Source: CAD feature listing. Evaluate the final solid. Frame: model axes, mm. Face numbers are marked on the shaded views. A direction names the side the tool comes from. Give positions to 0.01 mm unless a question says otherwise; leave off trailing zeros. Loops run counter-clockwise (first coordinate to the right, second up) from the corner with the lowest first, then second, coordinate; pieces in that order, holes last. Notation, with made-up numbers: (56, 28.25) - (94, 28.25) arc R28 cw to (94, 66.25) - close; hole circle Ø9 at (33.25, 81.25). An arc over 180 degrees is marked (long way). Put each result on its own line as item: value.
```python
from build123d import *

# Parameters (mm, degrees)
SKETCH1_W           = 205.38
SKETCH1_H           = 118.65
SKETCH1_W_2         = 189.38
SKETCH1_H_2         = 102.65
BOSS_EXTRUDE1_DEPTH = 13.5
SKETCH3_W           = 205.38
SKETCH3_H           = 118.65
BOSS_EXTRUDE2_DEPTH = 6.5
SKETCH4_R           = 2.5
CUT_EXTRUDE1_DEPTH  = 6
FILLET1_R           = 12.94


with BuildPart() as part:
    # Sketch1 → Boss-Extrude1 (new body)
    with BuildSketch(Plane(origin=(0, 0, 0), x_dir=(1, 0, 0), z_dir=(0, 1, 0))):
        Rectangle(SKETCH1_W, SKETCH1_H)
        Rectangle(SKETCH1_W_2, SKETCH1_H_2, mode=Mode.SUBTRACT)
    extrude(amount=BOSS_EXTRUDE1_DEPTH)

    # Sketch3 → Boss-Extrude2 (add)
    with BuildSketch(Plane(origin=(0, 13.5, 0), x_dir=(1, 0, 0), z_dir=(0, 1, 0))):
        Rectangle(SKETCH3_W, SKETCH3_H)
        Polygon((-94.69, 31.325), (-74.69, 51.325), (74.69, 51.325), (94.69, 31.325), (94.69, -31.325), (74.69, -51.325), (-74.69, -51.325), (-94.69, -31.325), align=None, mode=Mode.SUBTRACT)
    extrude(amount=BOSS_EXTRUDE2_DEPTH)

    # Sketch4 → Cut-Extrude1 (cut)
    with BuildSketch(Plane.XZ.offset(-13.5)):
        with Locations(Location((-88.94, 45.575, 0), (0, 0, 270))):
            Circle(SKETCH4_R)
        with Locations(Location((88.94, 45.575, 0), (0, 0, 90))):
            Circle(SKETCH4_R)
        with Locations(Location((88.94, -45.575, 0), (0, 0, 270))):
            Circle(SKETCH4_R)
        with Locations(Location((-88.94, -45.575, 0), (0, 0, 90))):
            Circle(SKETCH4_R)
    extrude(amount=-CUT_EXTRUDE1_DEPTH, mode=Mode.SUBTRACT)

    # Fillet1
    fillet1_edges = [part.edges().sort_by_distance(p)[0] for p in [
        (102.69, 10, 59.325),
        (-102.69, 10, 59.325),
        (-102.69, 10, -59.325),
        (102.69, 10, -59.325),
    ]]
    fillet(fillet1_edges, radius=FILLET1_R)


solid = part.part
```
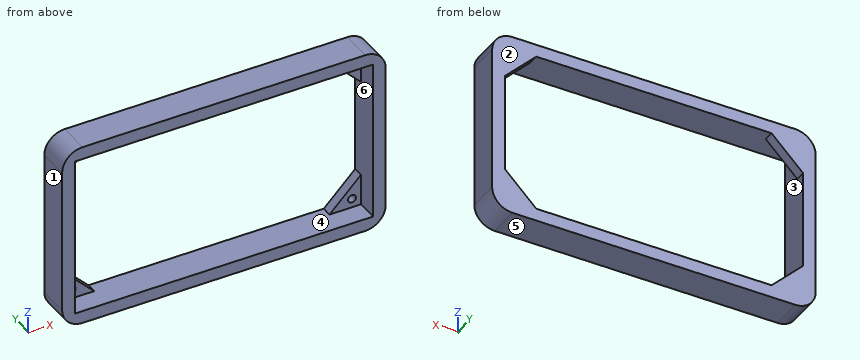
1) Section query C-C, the plane y = 15.75. Output: boundary loops of the cut face in (x, z) (3 decimals), plus the area to 3 significant figures.
Check result:
outline: (-102.69, -46.385) arc R12.94 ccw to (-89.75, -59.325) - (89.75, -59.325) arc R12.94 ccw to (102.69, -46.385) - (102.69, 46.385) arc R12.94 ccw to (89.75, 59.325) - (-89.75, 59.325) arc R12.94 ccw to (-102.69, 46.385) - close; hole (-94.69, -31.325) - (-74.69, -51.325) - (74.69, -51.325) - (94.69, -31.325) - (94.69, 31.325) - (74.69, 51.325) - (-74.69, 51.325) - (-94.69, 31.325) - close; hole circle Ø5 at (-88.94, -45.575); hole circle Ø5 at (-88.94, 45.575); hole circle Ø5 at (88.94, -45.575); hole circle Ø5 at (88.94, 45.575)
area: 5,510 mm²
2) Access query for the marked faces 5 and 6. Directions: +Z, -Z, +X, -X, +Y, -Y. A direction counts if a zero-diameter tool reaches every point of the face in a straight line with its end or side. Return the directions, or none.
Check result:
face 5: -Z, +X, -X, +Y, -Y
face 6: -Y
3) Material intervals for line 1 along Z through (x, y) = (-63.5, 12) (3 decimals); line 2 along X through (y, z) = (8.5, -4); line 3 along X through (y, z) = (18, 44.5) (3 decimals), sorted ascending. Write a range as [from, to].
Check result:
line 1: [-59.325, -51.325], [51.325, 59.325]
line 2: [-102.69, -94.69], [94.69, 102.69]
line 3: [-102.69, -91.197], [-86.683, -81.515], [81.515, 86.683], [91.197, 102.69]
4) Section query B-B, the plane x = -4. Output: boundary loops of the cut face in (y, z) (3 decimals), plus the area to 3 significant figures.
Check result:
outline: (0, -59.325) - (20, -59.325) - (20, -51.325) - (0, -51.325) - close; (0, 51.325) - (20, 51.325) - (20, 59.325) - (0, 59.325) - close
area: 320 mm²
5) Mould query, pull axis X, two halves, no side actions, for the marked faces 1, 2, 3 and 4. Classes: pulls with the +X half, pulls with the -X half, needs draft (parallel to the pull), parting line crosses it, or undercut.
Check result:
face 1: pulls with the -X half
face 2: needs draft
face 3: undercut
face 4: undercut
6) Section query A-A, the plane z = 5. Output: boundary loops of the cut face in (x, y).
Check result:
outline: (-102.69, 0) - (-94.69, 0) - (-94.69, 20) - (-102.69, 20) - close; (94.69, 0) - (102.69, 0) - (102.69, 20) - (94.69, 20) - close
7) Section query D-D, the plane z = -35.5. Output: boundary loops of the cut face in (x, y) (3 decimals), plus the area to 3 significant figures.
Check result:
outline: (-102.69, 0) - (-94.69, 0) - (-94.69, 13.5) - (-90.515, 13.5) - (-90.515, 20) - (-102.69, 20) - close; (90.515, 13.5) - (94.69, 13.5) - (94.69, 0) - (102.69, 0) - (102.69, 20) - (90.515, 20) - close
area: 374 mm²
8) Pin query (flat end, axial travel): P1, Ø4, axis at x = -89, z = 45.5, coming from the -Y side; P2, Ø6, axis at x = -88.94, z = -45.575, coming from the -Y side. Return the tip coordinate at first contact, or that it passes through.
Check result:
P1: y = 19.5
P2: y = 13.5
